from build123d import *

# Parameters (mm, degrees)
SKETCH2_R           = 0.85
BOSS_EXTRUDE1_DEPTH = 13.6


with BuildPart() as part:
    # Sketch2 → Boss-Extrude1 (new body)
    with BuildSketch(Plane.XY):
        Polygon((400, 0), (-400, 0), (-406.8, 0), (-406.8, 13.6), (-402.266666667, 13.6), (-306.362355233, 85.528233586), (-6.8, 310.200000045), (-6.8, 313.6), (0, 313.6), (800, 313.6), (806.8, 313.6), (806.8, 300), (802.266666606, 300), (406.8, 3.4), (406.8, 0), align=None)
        with Locations((0.107289977, 306.8)):
            Circle(SKETCH2_R, mode=Mode.SUBTRACT)
        with Locations((-399.99999994, 6.8)):
            Circle(SKETCH2_R, mode=Mode.SUBTRACT)
        with Locations((0, 6.8)):
            Circle(SKETCH2_R, mode=Mode.SUBTRACT)
        with Locations((400, 6.8)):
            Circle(SKETCH2_R, mode=Mode.SUBTRACT)
        with Locations((800, 306.8)):
            Circle(SKETCH2_R, mode=Mode.SUBTRACT)
        with Locations((400, 306.8)):
            Circle(SKETCH2_R, mode=Mode.SUBTRACT)
        Polygon((-6.8, 13.6), (-6.8, 293.200000044), (-298.202355233, 74.648233587), (-379.600000002, 13.6), align=None, mode=Mode.SUBTRACT)
        Polygon((6.8, 300), (6.8, 20.4), (106.280361955, 95.010271466), (379.6, 300), align=None, mode=Mode.SUBTRACT)
        Polygon((393.2, 13.6), (393.2, 293.2), (114.440361955, 84.130271466), (20.4, 13.6), align=None, mode=Mode.SUBTRACT)
        Polygon((406.8, 20.400000001), (406.8, 300), (779.599999942, 300), align=None, mode=Mode.SUBTRACT)
    extrude(amount=BOSS_EXTRUDE1_DEPTH)


solid = part.part
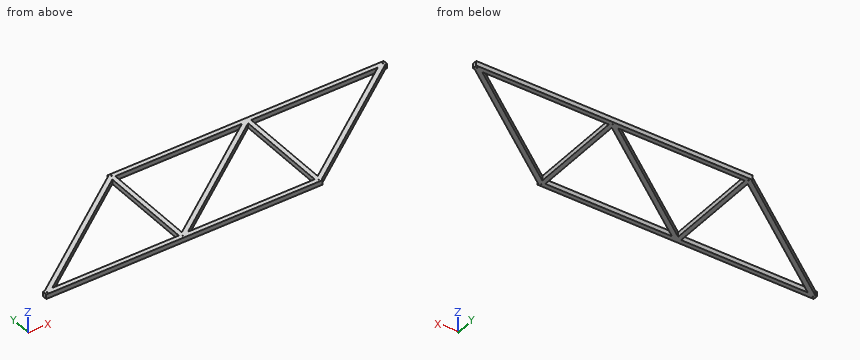
Read the model definition and answer for the solid it produces. Units are mm, in the model's axes. Round coordinates to 2 decimals unless told otherwise and drop trailing zeros. Order: outer loops, then holes, each group sorted by start corner. A loop starts at its lowest first (then second) coordinate and runs counter-clockwise, first axis right, second up.
1) Straight lines are drawn through the part: L1, parallel to Y at x = 400, z = 9.5; L2, parallel to X at y = 306.8, z = 9.25; L3, parallel to X at y = 97.5, z = 1.75. For each, find the intervals that lie inside material, in ascending order.
2) Flat-ended cylindrical pins translate along their axes: pin 1 (5 mm diameter, centred on y = 188.5, z = 2.5, fed in from -X); pin 2 (2 mm diameter, centred on x = 400, y = 306.8, fed in from -Z); pin 3 (1.5 mm diameter, centred on y = 186.5, z = 6.5, fed in from +X); pin 4 (4 mm diameter, centred on y = 200.5, z = 3, fed in from +X). Find the tip coordinate at first contact, or state that the pin passes through.
3) The part is cut by section A-A on x = 573. Write down the section's boundary in (y, z).
4) The part is cut by section D-D on z = 10.5. Give the number of separate pieces and of enclosed holes in the cut face, plus the area to 3 significant figures.
5) The part is cut by section C-C on x = 86. Write down the section's boundary in (y, z), plus the area to 3 significant figures.
6) The part is cut by section B-B on y = 184.5. Write down the section's boundary in (x, z).
Resolved:
1. L1: y = 0 to 5.95, 7.65 to 305.95, 307.65 to 313.6
1. L2: x = -11.33 to -0.74, 0.96 to 399.15, 400.85 to 799.15, 800.85 to 806.8
1. L3: x = -290.4 to -267.73, -6.8 to 6.8, 109.6 to 132.27, 393.2 to 406.8, 509.6 to 532.27
2. pin 1: stops at x = -172.4
2. pin 2: stops at z = 0
2. pin 3: stops at x = 651.93
2. pin 4: stops at x = 672.27
3. outline: (128.05, 0) - (145.05, 0) - (145.05, 13.6) - (128.05, 13.6) - close; (300, 0) - (313.6, 0) - (313.6, 13.6) - (300, 13.6) - close
4. separate pieces: 1
4. enclosed holes: 10
4. area: 49,400 mm2
5. outline: (0, 0) - (13.6, 0) - (13.6, 13.6) - (0, 13.6) - close; (62.8, 0) - (79.8, 0) - (79.8, 13.6) - (62.8, 13.6) - close; (300, 0) - (313.6, 0) - (313.6, 13.6) - (300, 13.6) - close
5. area: 601 mm2
6. outline: (-174.4, 0) - (-151.73, 0) - (-151.73, 13.6) - (-174.4, 13.6) - close; (-6.8, 0) - (6.8, 0) - (6.8, 13.6) - (-6.8, 13.6) - close; (225.6, 0) - (248.27, 0) - (248.27, 13.6) - (225.6, 13.6) - close; (393.2, 0) - (406.8, 0) - (406.8, 13.6) - (393.2, 13.6) - close; (625.6, 0) - (648.27, 0) - (648.27, 13.6) - (625.6, 13.6) - close
